from build123d import *

# Parameters (mm, degrees)
SKETCH1_W             = 10
SKETCH1_H             = 13.5
SKETCH1_W_2           = 7.3
SKETCH1_H_2           = 10.5
BOSS_EXTRUDE1_DEPTH   = 15
SKETCH1_3_W           = 0.5
SKETCH1_3_H           = 10.5
BOSS_EXTRUDE2_DEPTH   = 6.5
BOSS_EXTRUDE3_DEPTH   = 5
F_6_CLEARANCE_HOLE1_D = 3.7973
SKETCH5_W             = 6.3
SKETCH5_H             = 10.5
SKETCH5_W_2           = 4.3
SKETCH5_H_2           = 8.5
BOSS_EXTRUDE4_DEPTH   = 1.5
FILLET1_R             = 2
FILLET2_SIZE          = 1
FILLET3_R             = 1


with BuildPart() as part:
    # Sketch1 → Boss-Extrude1 (new body)
    with BuildSketch(Plane(origin=(0, 0, 0), x_dir=(1, 0, 0), z_dir=(0, 1, 0))):
        Rectangle(SKETCH1_W, SKETCH1_H)
        Rectangle(SKETCH1_W_2, SKETCH1_H_2, mode=Mode.SUBTRACT)
    extrude(amount=BOSS_EXTRUDE1_DEPTH)

    # Sketch1<3> → Boss-Extrude2 (add)
    with BuildSketch(Plane(origin=(0, 0, 0), x_dir=(1, 0, 0), z_dir=(0, 1, 0))):
        with Locations((-3.4, 0)):
            Rectangle(SKETCH1_3_W, SKETCH1_3_H)
        with Locations((3.4, 0)):
            Rectangle(SKETCH1_3_W, SKETCH1_3_H)
    extrude(amount=BOSS_EXTRUDE2_DEPTH)

    # Sketch2 → Boss-Extrude3 (add)
    with BuildSketch(Plane.XY.offset(6.75)):
        with BuildLine():
            ThreePointArc((13, 13), (12.414213562, 14.414213562), (11, 15))
            Line((11, 15), (5, 15))
            Line((5, 15), (5, 7))
            Line((5, 7), (11, 7))
            ThreePointArc((11, 7), (12.414213562, 7.585786438), (13, 9))
            Line((13, 9), (13, 13))
        make_face()
        with BuildLine():
            Line((-13, 9), (-13, 13))
            ThreePointArc((-13, 13), (-12.414213562, 14.414213562), (-11, 15))
            Line((-11, 15), (-5, 15))
            Line((-5, 15), (-5, 7))
            Line((-5, 7), (-11, 7))
            ThreePointArc((-11, 7), (-12.414213562, 7.585786438), (-13, 9))
        make_face()
    extrude(amount=-BOSS_EXTRUDE3_DEPTH)

    # #6 Clearance Hole1 (through all)
    with Locations(Plane.XY.offset(6.75)):
        with Locations((-9, 11), (9, 11)):
            Hole(F_6_CLEARANCE_HOLE1_D / 2)

    # Sketch5 → Boss-Extrude4 (add)
    with BuildSketch(Plane.XZ):
        Rectangle(SKETCH5_W, SKETCH5_H)
        Rectangle(SKETCH5_W_2, SKETCH5_H_2, mode=Mode.SUBTRACT)
    extrude(amount=-BOSS_EXTRUDE4_DEPTH)

    # Fillet1
    fillet1_edges = [part.edges().sort_by_distance(p)[0] for p in [
        (-5, 7.5, -6.75),
        (5, 7.5, -6.75),
    ]]
    fillet(fillet1_edges, radius=FILLET1_R)

    # Fillet2
    fillet2_edges = [part.edges().sort_by_distance(p)[0] for p in [
        (0, 1.5, -4.25),
        (2.15, 1.5, 0),
        (0, 1.5, 4.25),
        (-2.15, 1.5, 0),
    ]]
    chamfer(fillet2_edges, length=FILLET2_SIZE - 0.0001)  # a hair under: the kernel refuses the full size

    # Fillet3
    fillet3_edges = [part.edges().sort_by_distance(p)[0] for p in [
        (0, 0, -6.75),
        (0, 15, -6.75),
        (5, 0, 1),
        (-5, 0, 1),
        (-4.414213562, 0, -6.164213562),
        (4.414213562, 0, -6.164213562),
        (5, 15, -1.5),
        (-5, 15, -1.5),
        (-4.414213562, 15, -6.164213562),
        (4.414213562, 15, -6.164213562),
        (8, 7, 1.75),
        (8, 15, 1.75),
        (12.414213562, 14.414213562, 1.75),
        (13, 11, 1.75),
        (12.414213562, 7.585786438, 1.75),
        (-12.414213562, 7.585786438, 1.75),
        (-13, 11, 1.75),
        (-12.414213562, 14.414213562, 1.75),
        (-8, 15, 1.75),
        (-8, 7, 1.75),
    ]]
    fillet(fillet3_edges, radius=FILLET3_R)


solid = part.part
The listing builds one solid part. Answer for the finished solid, in the listing's coordinates (mm). A direction names the side the tool comes from. Coordinates: 2 decimals unless noted, no trailing zeros. Write each loop counter-clockwise with the first axis right and the second up, starting at its lowest first coordinate (ties: lowest second). Pieces come first, ordered by that corner, then holes. Notation, with made-up numbers: (39.25, 83.5) - (53.25, 83.5) arc R15 cw to (53.25, 97.5) - close; hole circle Ø1 at (42.25, 86.25). An arc over 180 degrees is marked (long way). Put each result on its own line as item: value.
1. Flat-ended cylindrical pins translate along their axes: pin 1 Ø1.8 at (x, y) = (-7.5, 11.5) entering from -Z; pin 2 Ø4.5 at (x, z) = (8.5, 4) entering from -Y; pin 3 Ø1.5 at (x, z) = (2, -3) entering from +Y. Find the tip coordinate at first contact, or state that the pin passes through.
Answer sheet:
pin 1: stops at z = 1.75
pin 2: stops at y = 7
pin 3: stops at y = 1.1
2. A tool of negligible diameter and unlimited length cuts with its end or side. For faces 1 (the face through (6.9, 11, 1.75)), 2 (the face through (8, 7, 5)), 3 (the face through (-6.9, 11, 1.75)), 4 (the face through (-0.04, 1.01, 4.76)), 5 (the face through (-8, 7, 5)), from which of +Z, -Z, +X, -X, +Y, -Y can it reach the whole face along a straight path? Write none if from no direction.
Answer sheet:
face 1: -Z, +X, +Y, -Y
face 2: +Z, -Z, +X, -Y
face 3: -Z, -X, +Y, -Y
face 4: +Y
face 5: +Z, -Z, -X, -Y
3. The part is cut by section A-A on y = 11. Give the vertices of the cut face in (x, z), plus the area to 3 significant figures.
Answer sheet:
outline: (-13, 2.75) arc R1 ccw to (-12, 1.75) - (-10.9, 1.75) - (-10.9, 6.75) - (-13, 6.75) - close; (-7.1, 1.75) - (-5, 1.75) - (-5, -4.75) arc R2 ccw to (-3, -6.75) - (3, -6.75) arc R2 ccw to (5, -4.75) - (5, 1.75) - (7.1, 1.75) - (7.1, 6.75) - (-7.1, 6.75) - close; (10.9, 1.75) - (12, 1.75) arc R1 ccw to (13, 2.75) - (13, 6.75) - (10.9, 6.75) - close; hole (-3.65, -5.25) - (3.65, -5.25) - (3.65, 5.25) - (-3.65, 5.25) - close
area: 98.2 mm^2
4. Determine the mould class of faces 6 (the face through (-8.753, 12.882, 4.215)), 7 (the face through (2.66, 1.01, -0.07)), 8 (the face through (0, 8, -5.25)), 9 (the face through (0.042, 14.699, -6.465)) for opening direction Z: pulls with the +Z half, pulls with the -Z half, needs draft (parallel to the pull), parting line crosses it, or undercut.
Answer sheet:
face 6: needs draft
face 7: undercut
face 8: undercut
face 9: pulls with the -Z half
5. Find the intervals of material crossed by line 1 along Y through (x, z) = (9, 3.15); line 2 along X through (y, z) = (4.75, 5); line 3 along X through (y, z) = (6.75, 0.25), in increasing order. Write a range as from..to.
Answer sheet:
line 1: y = 7..9.1, 12.9..15
line 2: x = -5..-3.15, 3.15..5
line 3: x = -5..-3.65, 3.65..5
6. The part is cut by section D-D on z = 5.75. Give the vertices of the cut face in (x, y).
Answer sheet:
outline: (-13, 9) arc R2 ccw to (-11, 7) - (-5, 7) - (-5, 1) arc R1 ccw to (-4, 0) - (4, 0) arc R1 ccw to (5, 1) - (5, 7) - (11, 7) arc R2 ccw to (13, 9) - (13, 13) arc R2 ccw to (11, 15) - (-11, 15) arc R2 ccw to (-13, 13) - close; hole circle Ø3.8 at (-9, 11); hole circle Ø3.8 at (9, 11)
7. The part is cut by section B-B on x = -9. Give the vertices of the cut face in (y, z).
Answer sheet:
outline: (7, 2.75) arc R1 ccw to (8, 1.75) - (9.1, 1.75) - (9.1, 6.75) - (7, 6.75) - close; (12.9, 1.75) - (14, 1.75) arc R1 ccw to (15, 2.75) - (15, 6.75) - (12.9, 6.75) - close
